Verification items for this drawing (mm, ordinates from the low corner). A direction names the side the tool comes from. Give positions to 0.01 mm unless a question says otherwise; leave off trailing zeros. Write each loop counter-clockwise with the first axis right and the second up, starting at its lowest first coordinate (ties: lowest second). Pieces come first, ordered by that corner, then holes. Notation, with made-up numbers: (60.5, -23) -> (86.5, -23) arc R19 cw to (86.5, -14) -> close; hole circle Ø1 at (-30.5, -37.75). An arc over 180 degrees is marked (long way). Answer as a JSON object with one key per item and string values.
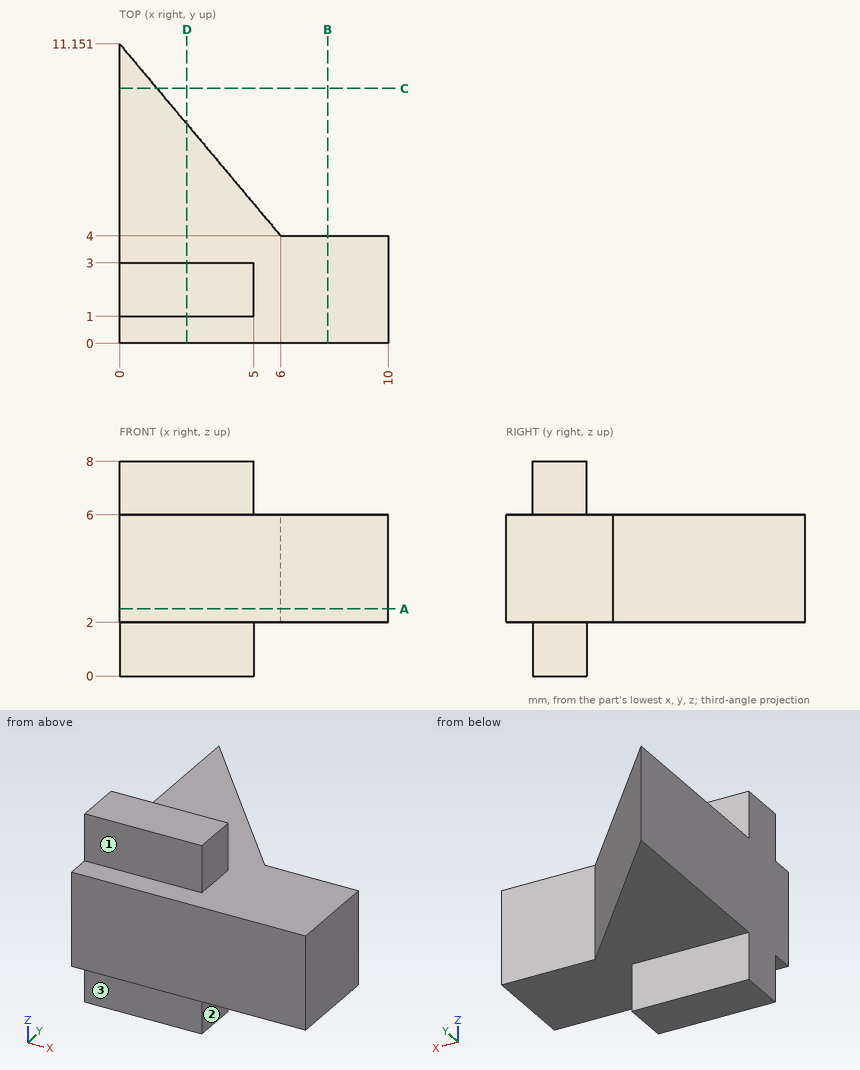
1. Go/stop test with flat-tipped pins: P1, Ø1, axis at x = 1.5, z = 1, coming from the -Y side; P2, Ø1, axis at x = 3, z = 0.5, coming from the +Y side; P3, Ø2, axis at x = 7.5, z = 4, coming from the +Y side. Record where each tip stops, or that it passes through.
Determined:
{"P1": "y = 1", "P2": "y = 3", "P3": "y = 4"}
2. Sectioned sample at C-C, the plane y = 9.5. Enter the section's corners in (x, z) (1 decimal).
Determined:
{"outline": "(0, 2) -> (1.4, 2) -> (1.4, 6) -> (0, 6) -> close"}
3. Sectioned sample at D-D, the plane x = 2.5. Enter the section's corners in (y, z), plus the area to 3 significant figures.
Determined:
{"outline": "(0, 2) -> (1, 2) -> (1, 0) -> (3, 0) -> (3, 2) -> (8.17, 2) -> (8.17, 6) -> (3, 6) -> (3, 8) -> (1, 8) -> (1, 6) -> (0, 6) -> close", "area": "40.7 mm^2"}
4. Sectioned sample at B-B, the plane x = 7.75. Enter the section's corners in (y, z), plus the area to 3 significant figures.
Determined:
{"outline": "(0, 2) -> (4, 2) -> (4, 6) -> (0, 6) -> close", "area": "16.0 mm^2"}
5. Scan lines: L1, parallel to Y at x = 3.25, z = 7; L2, parallel to Z at x = 2, y = 3.5; L3, parallel to X at y = 7.75, z = 5 (1 decimal). Record each from-to range of solid material in increasing order. Write a range as [from, to].
Determined:
{"L1": "[1, 3]", "L2": "[2, 6]", "L3": "[0, 2.9]"}
6. Access from +Z, -Z, +X, -X, +Y, -Y to the whole of each face (thin tool, end or side, straight path). Record for the marked faces 1, 2 and 3.
Determined:
{"face 1": "+Z, +X, -X, -Y", "face 2": "-Z, +X, +Y, -Y", "face 3": "-Z, +X, -X, -Y"}
7. Sectioned sample at A-A, the plane z = 2.5. Enter the section's corners in (x, y).
Determined:
{"outline": "(0, 0) -> (10, 0) -> (10, 4) -> (6, 4) -> (0, 11.15) -> close"}
